```python
from build123d import *

# Parameters (mm, degrees)
BOSS_EXTRUDE1_DEPTH = 60
CUT_EXTRUDE1_DEPTH  = 5


with BuildPart() as part:
    # Sketch1 → Boss-Extrude1 (new body)
    with BuildSketch(Plane(origin=(0, 0, 0), x_dir=(1, 0, 0), z_dir=(0, 1, 0))):
        Polygon((-32.5, -30.12), (-32.5, -33.12), (-58.915, -33.12), (-58.915, 33.12), (58.915, 33.12), (58.915, -33.12), (32.5, -33.12), (32.5, -30.12), (55.915, -30.12), (55.915, 30.12), (-55.915, 30.12), (-55.915, -30.12), align=None)
    extrude(amount=BOSS_EXTRUDE1_DEPTH)

    # Sketch2 → Cut-Extrude1 (cut)
    with BuildSketch(Plane(origin=(0, 60, 0), x_dir=(1, 0, 0), z_dir=(0, 1, 0))):
        Polygon((-34.7, -30.62), (-34.7, -31.82), (-58.115, -31.82), (-58.115, 31.82), (58.115, 31.82), (58.115, -31.82), (34.7, -31.82), (34.7, -30.62), (56.915, -30.62), (56.915, 30.62), (-56.915, 30.62), (-56.915, -30.62), align=None)
    extrude(amount=-CUT_EXTRUDE1_DEPTH, mode=Mode.SUBTRACT)


solid = part.part
```
The listing builds one solid part. Answer for the finished solid, in the listing's coordinates (mm). A direction names the side the tool comes from. Coordinates: 2 decimals unless noted, no trailing zeros. Write each loop counter-clockwise with the first axis right and the second up, starting at its lowest first coordinate (ties: lowest second). Pieces come first, ordered by that corner, then holes. Notation, with made-up numbers: M -15,19.25 L -2,19.25 A16 cw -2,39.25 Z; hole C 63.25,10 d6. An arc over 180 degrees is marked long. Use a Markdown table: item, result. Add a question column.
1. Section B-B (x = -46.5) is taken. Give the vertices of the cut face in (y, z), plus the area to 3 significant figures.
2. For a pull along Z with two mould halves and no side action, classify faces 6 (the flat face through (-46, 30, 33.12)), 7 (the flat face through (-46, 58, 31.82)), 8 (the flat face through (-26, 60, -32)) as +Z half, -Z half, draft (parallel to the pull), parting line (faces both ways), or undercut.
3. Straight lines are drawn through the part: line 1 along X through (y, z) = (47.5, -6.5) (3 decimals); line 2 along Z through (x, y) = (48.5, 49); line 3 along Z through (x, y) = (16.5, 39.5). For each, find the intervals that lie inside material, in ascending order. Write a range as [from, to].
4. Section C-C (y = 53) is taken. Give the vertices of the cut face in (x, z) (3 decimals), plus the area to 3 significant figures.
5. Section D-D (x = 31) is taken. Give the vertices of the cut face in (y, z).
6. Given P1, Ø5.5, axis at x = 0, y = 57.5, coming from the +Z side, flat-ended and moving along its own axis, determine where the tip first touches the part or whether it passes through.
7. Section A-A (z = -23) is taken. Give the vertices of the cut face in (x, y) (3 decimals), plus the area to 3 significant figures.
8. Which of the six approach directions +Z, -Z, +X, -X, +Y, -Y give full straight-line access (tool end or side, diameter ignored) to faces 1 (the flat face through (46, 58, 30.62)), 2 (the flat face through (0, 0, -32)), 3 (the flat face through (-58.915, 30, 0)), 4 (the flat face through (-44, 30, 30.12)), 5 (the flat face through (32.5, 30, 32))?
Data:
| question | item | result |
|---|---|---|
| 1 | outline | M 0,-33.12 L 60,-33.12 L 60,-31.82 L 55,-31.82 L 55,-30.62 L 60,-30.62 L 60,-30.12 L 0,-30.12 Z; M 0,30.12 L 60,30.12 L 60,30.62 L 55,30.62 L 55,31.82 L 60,31.82 L 60,33.12 L 0,33.12 Z |
| 1 | area | 348 mm2 |
| 2 | face 6 | +Z half |
| 2 | face 7 | undercut |
| 2 | face 8 | draft |
| 3 | line 1 | x = [-58.915, -55.915], [55.915, 58.915] |
| 3 | line 2 | z = [-33.12, -30.12], [30.12, 33.12] |
| 3 | line 3 | z = [-33.12, -30.12] |
| 4 | outline | M -58.915,-33.12 L 58.915,-33.12 L 58.915,33.12 L 32.5,33.12 L 32.5,30.12 L 55.915,30.12 L 55.915,-30.12 L -55.915,-30.12 L -55.915,30.12 L -32.5,30.12 L -32.5,33.12 L -58.915,33.12 Z |
| 4 | area | 873 mm2 |
| 5 | outline | M 0,-33.12 L 60,-33.12 L 60,-31.82 L 55,-31.82 L 55,-30.62 L 60,-30.62 L 60,-30.12 L 0,-30.12 Z |
| 6 | P1 | stops at z = -30.12 |
| 7 | outline | M -58.915,0 L -55.915,0 L -55.915,60 L -56.915,60 L -56.915,55 L -58.115,55 L -58.115,60 L -58.915,60 Z; M 55.915,0 L 58.915,0 L 58.915,60 L 58.115,60 L 58.115,55 L 56.915,55 L 56.915,60 L 55.915,60 Z |
| 7 | area | 348 mm2 |
| 8 | face 1 | +Y |
| 8 | face 2 | +Z, -Z, +X, -X, -Y |
| 8 | face 3 | +Z, -Z, -X, +Y, -Y |
| 8 | face 4 | +Y, -Y |
| 8 | face 5 | +Z, +Y, -Y |
